Input: part model. Units: mm. Frame: model coordinates. A direction names the side the tool comes from. Coordinates: 2 decimals unless noted, no trailing zeros. Write each loop counter-clockwise with the first axis right and the second up, starting at its lowest first coordinate (ties: lowest second). Pieces come first, ordered by that corner, then holes. Notation, with made-up numbers: (0, -0.5) - (38, -0.5) arc R22 ccw to (38, 38.5) - close; hole circle Ø2 at (17, 18.25). An arc over 180 degrees is marked (long way). One line per question, with ' | ' between items. Start each with the question number.
1) Line query: line 1 (Y direction, x = 11.5, z = 1.9); line 2 (X direction, y = -5.5, z = 0.1); line 3 (X direction, y = -72.5, z = 0.55). Output: solid intervals per line, ascending.
2) Draft query along X for faces 6 (the flat face through (17, -56.2, 1)), 7 (the flat face through (15, -2, 1)), 8 (the flat face through (0, -71, 1)), 9 (the flat face through (29.7, -17, 1)). Return one class per face: released by +X, released by -X, zero draft, split by the parting line, or undercut.
3) Reachability of faces 1 (the flat face through (1, -25.1, 1)), 2 (the flat face through (3, -28, 1)), 3 (the flat face through (31.2, -7, 1)), 4 (the flat face through (30, -53.3, 1)), 5 (the flat face through (2.8, -44.8, 0)) from +Z, -Z, +X, -X, +Y, -Y: full face, straight path, thin tool, end or side. Return the list, or none.
4) Section query A-A on y = -22. Return loops of the section in (x, z), and give its area (3 significant figures).
5) Section query D-D on y = -34.5. Return loops of the section in (x, z), and give its area (3 significant figures).
6) Section query B-B on x = 21. Return loops of the section in (y, z), and give its area (3 significant figures).
7) Section query C-C on z = 1.25. Give the number of separate pieces and of enclosed holes in the cut face, and give its area (3 significant figures).
8) First-contact query: P1, Ø1, axis at y = -63.5, z = 1, coming from the -X side; P2, Ø0.8, axis at x = 1, z = 0.5, coming from the -Y side; P3, Ø0.6, axis at y = -64, z = 0.5, coming from the +X side. Flat tips, straight axial feed; report the tip coordinate or a pass-through.
```python
from build123d import *

# Parameters (mm, degrees)
SKETCH_W        = 31.2
SKETCH_H        = 78.4
SKETCH_W_2      = 25.2
SKETCH_H_2      = 52.2
SKETCH_W_3      = 18.2
SKETCH_H_3      = 18.2
PAD_DEPTH       = 2
SKETCH007_W     = 11.282879
SKETCH007_H     = 15.2
SKETCH007_W_2   = 12.568334
SKETCH007_W_3   = 28.383078
SKETCH007_W_4   = 31.922889
POCKET002_DEPTH = 5
FILLET002_R     = 4


with BuildPart() as part:
    # Sketch → Pad (new body)
    with BuildSketch(Plane.XY):
        with Locations((15.6, -39.2)):
            Rectangle(SKETCH_W, SKETCH_H)
        with Locations((15.6, -28.1)):
            Rectangle(SKETCH_W_2, SKETCH_H_2, mode=Mode.SUBTRACT)
        with Locations((17.1, -65.3)):
            Rectangle(SKETCH_W_3, SKETCH_H_3, mode=Mode.SUBTRACT)
    extrude(amount=PAD_DEPTH)

    # Sketch007 (on Face13 of Pad) → Pocket002 (cut)
    with BuildSketch(Plane(origin=(0, 0, 0), x_dir=(1, 0, 0), z_dir=(0, 0, -1))):
        with Locations((-4.141439, 60.9)):
            Rectangle(SKETCH007_W, SKETCH007_H)
        with Locations((-4.784167, 17.5)):
            Rectangle(SKETCH007_W_2, SKETCH007_H)
        with Locations((43.891539, 60.9)):
            Rectangle(SKETCH007_W_3, SKETCH007_H)
        with Locations((45.661445, 17.5)):
            Rectangle(SKETCH007_W_4, SKETCH007_H)
    extrude(amount=-POCKET002_DEPTH, mode=Mode.SUBTRACT)

    # Fillet002
    fillet002_edges = [part.edges().sort_by_distance(p)[0] for p in [
        (31.2, 0, 1),
        (0, 0, 1),
        (0, -78.4, 1),
        (31.2, -78.4, 1),
    ]]
    fillet(fillet002_edges, radius=FILLET002_R)


solid = part.part
```
Answer key:
1) line 1: -78.4 to -74.4, -56.2 to -54.2, -2 to 0 | line 2: 0 to 3, 28.2 to 31.2 | line 3: 0 to 8, 26.2 to 31.2
2) face 6: undercut | face 7: undercut | face 8: released by -X | face 9: released by +X
3) face 1: +Z, -Z, -X | face 2: +Z, -Z | face 3: +Z, -Z, +X, +Y, -Y | face 4: +Z, -Z, +X | face 5: -Z, +X, -X, +Y, -Y
4) outline: (1.5, 0) - (3, 0) - (3, 2) - (1.5, 2) - close; (28.2, 0) - (29.7, 0) - (29.7, 2) - (28.2, 2) - close | area: 6.00 mm²
5) outline: (0, 0) - (3, 0) - (3, 2) - (0, 2) - close; (28.2, 0) - (31.2, 0) - (31.2, 2) - (28.2, 2) - close | area: 12.0 mm²
6) outline: (-78.4, 0) - (-74.4, 0) - (-74.4, 2) - (-78.4, 2) - close; (-56.2, 0) - (-54.2, 0) - (-54.2, 2) - (-56.2, 2) - close; (-2, 0) - (0, 0) - (0, 2) - (-2, 2) - close | area: 16.0 mm²
7) separate pieces: 1 | enclosed holes: 2 | area: 694 mm²
8) P1: x = 1.5 | P2: y = -77.44 | P3: x = 29.7
